Could you check a few things on this model? Use its own coordinates, in mm. Face numbers are marked on the shaded views. A direction names the side the tool comes from. Round coordinates to 2 decimals unless told otherwise and drop trailing zeros. Write each loop counter-clockwise with the first axis right and the second up, starting at its lowest first coordinate (ties: lowest second). Pieces come first, ordered by that corner, then holes. Notation, with made-up numbers: (-19.75, -34) -> (39.25, -34) arc R19 cw to (39.25, 2) -> close; hole circle Ø8 at (57, -35). An arc over 180 degrees is marked (long way). One line per question, with ' | ' between items. Start each with the question number.
1. For the marked faces 5, 6 and 7, which set-ups out of +Z, -Z, +X, -X, +Y, -Y let a thin tool reach every point of the face, with its end or its side?
2. Imagine slicing it at D-D, the plane y = 18.5. List the corners of the cut face in (x, z) for me, and give its area (3 significant figures).
3. Thinking about a two-plate mould opening in Z: for the marked faces 1, 2, 3 and 4, which applies, released by +Z, released by -Z, zero draft, split by the parting line, or undercut?
4. Imagine slicing it at C-C, the plane x = -19. List the corners of the cut face in (y, z) for me.
5. Imagine slicing it at B-B, the plane z = 6.5. State how many separate pieces and enclosed holes the cut face has, and give its area (3 significant figures).
6. For pin 1 Ø5.5 at (x, z) = (-19.5, 8) entering from +Y; pin 2 Ø3 at (x, z) = (5, 7.5) entering from +Y; pin 3 Ø5 at (x, y) = (0, -5) entering from +Z, each with a flat end and sliding along its axis, tell me the tip position at first contact or that it passes through.
7. If I drill on line 1 along Y through (x, z) = (0, 7); line 2 along Y through (x, z) = (0, 14.35); line 3 along X through (y, z) = (6.5, 10.25), over which ranges is the centre line in solid material (lowest first)? Write a range as [from, to].
8. Imagine slicing it at A-A, the plane y = -23.5. List the corners of the cut face in (x, z) for me.
from build123d import *

# Parameters (mm, degrees)
BOSS_EXTRUDE1_DEPTH = 15
CUT_EXTRUDE1_REACH  = 57
SKETCH2_R           = 2.25
SKETCH3_R           = 5.54
CUT_EXTRUDE2_DEPTH  = 21
SKETCH4_W           = 24
SKETCH4_H           = 7
CUT_EXTRUDE3_DEPTH  = 29
CUT_EXTRUDE4_REACH  = 17
CUT_EXTRUDE5_DEPTH  = 1.5
SKETCH7_R           = 3.25
BOSS_EXTRUDE2_DEPTH = 13.5
CUT_EXTRUDE6_REACH  = 15.5
SKETCH8_R           = 1.5
SKETCH9_R           = 2.5
CUT_EXTRUDE7_DEPTH  = 12
SKETCH10_R          = 0.48
BOSS_EXTRUDE3_DEPTH = 1.5


with BuildPart() as part:
    # Sketch1 → Boss-Extrude1 (new body)
    with BuildSketch(Plane.XY):
        with BuildLine():
            Line((25, 0), (25, -30))
            Line((25, -30), (-25, -30))
            Line((-25, -30), (-25, 0))
            ThreePointArc((-25, 0), (0, 25), (25, 0))
        make_face()
    extrude(amount=BOSS_EXTRUDE1_DEPTH)

    # Sketch2 → Cut-Extrude1 (cut, up to next)
    with BuildSketch(Plane.XZ.offset(30), mode=Mode.PRIVATE) as cut_extrude1_sk1:
        with Locations((-19, 7.5)):
            Circle(SKETCH2_R)
    cut_extrude1_tool1 = extrude(cut_extrude1_sk1.sketch, amount=-CUT_EXTRUDE1_REACH, mode=Mode.PRIVATE) & part.part
    add(cut_extrude1_tool1.solids().sort_by_distance((-19, -30, 7.5))[0], mode=Mode.SUBTRACT)
    # Sketch2 → Cut-Extrude1 (cut, up to next)
    with BuildSketch(Plane.XZ.offset(30), mode=Mode.PRIVATE) as cut_extrude1_sk2:
        with Locations((19, 7.5)):
            Circle(SKETCH2_R)
    cut_extrude1_tool2 = extrude(cut_extrude1_sk2.sketch, amount=-CUT_EXTRUDE1_REACH, mode=Mode.PRIVATE) & part.part
    add(cut_extrude1_tool2.solids().sort_by_distance((19, -30, 7.5))[0], mode=Mode.SUBTRACT)

    # Sketch3 → Cut-Extrude2 (cut)
    with BuildSketch(Plane(origin=(0, 24.127056635, 0), x_dir=(1, 0, 0), z_dir=(0, 1, 0))):
        with Locations((19, -7.5)):
            Circle(SKETCH3_R)
        with Locations((-19, -7.5)):
            Circle(SKETCH3_R)
    extrude(amount=-CUT_EXTRUDE2_DEPTH, mode=Mode.SUBTRACT)

    # Sketch4 → Cut-Extrude3 (cut)
    with BuildSketch(Plane.XZ.offset(30)):
        with Locations((0, 7.5)):
            Rectangle(SKETCH4_W, SKETCH4_H)
    extrude(amount=-CUT_EXTRUDE3_DEPTH, mode=Mode.SUBTRACT)

    # Sketch5 → Cut-Extrude4 (cut, up to next)
    with BuildSketch(Plane.XY.offset(15), mode=Mode.PRIVATE) as cut_extrude4_sk1:
        with BuildLine():
            Line((11.251747285, -5), (15, -5))
            ThreePointArc((15, -5), (0, -20), (-15, -5))
            ThreePointArc((-15, -5), (-13.858192988, 0.740251485), (-10.606601718, 5.606601718))
            Line((-10.606601718, 5.606601718), (-7.956186805, 2.956186805))
            ThreePointArc((-7.956186805, 2.956186805), (-10.395259022, -0.694142729), (-11.251747285, -5))
            ThreePointArc((-11.251747285, -5), (0, -16.251747285), (11.251747285, -5))
        make_face()
    cut_extrude4_tool1 = extrude(cut_extrude4_sk1.sketch, amount=-CUT_EXTRUDE4_REACH, mode=Mode.PRIVATE) & part.part
    add(cut_extrude4_tool1.solids().sort_by_distance((13.125874, -5.394423, 15))[0], mode=Mode.SUBTRACT)

    # Sketch6 → Cut-Extrude5 (cut)
    with BuildSketch(Plane.XY.offset(15)):
        with BuildLine():
            Line((0.541549319, -1.795436951), (14.169837516, 1.800031788))
            ThreePointArc((14.169837516, 1.800031788), (16.028383105, 0.812877901), (15.18982596, -1.117274015))
            Line((15.18982596, -1.117274015), (2.352905683, -7.241948894))
            ThreePointArc((2.352905683, -7.241948894), (-3.083924533, -6.02562638), (0.541549319, -1.795436951))
        make_face()
    extrude(amount=-CUT_EXTRUDE5_DEPTH, mode=Mode.SUBTRACT)

    # Sketch7 → Boss-Extrude2 (add)
    with BuildSketch(Plane.XY.offset(13.5)):
        with Locations((0, -5)):
            Circle(SKETCH7_R)
    extrude(amount=-BOSS_EXTRUDE2_DEPTH)

    # Sketch8 → Cut-Extrude6 (cut, up to next)
    with BuildSketch(Plane.XY.offset(13.5), mode=Mode.PRIVATE) as cut_extrude6_sk1:
        with Locations((0, -5)):
            Circle(SKETCH8_R)
    cut_extrude6_tool1 = extrude(cut_extrude6_sk1.sketch, amount=-CUT_EXTRUDE6_REACH, mode=Mode.PRIVATE) & part.part
    add(cut_extrude6_tool1.solids().sort_by_distance((0, -5, 13.5))[0], mode=Mode.SUBTRACT)

    # Sketch9 → Cut-Extrude7 (cut)
    with BuildSketch(Plane(origin=(0, 0, 0), x_dir=(-1, 0, 0), z_dir=(0, 0, -1))):
        with Locations((0, -5)):
            Circle(SKETCH9_R)
    extrude(amount=-CUT_EXTRUDE7_DEPTH, mode=Mode.SUBTRACT)

    # Sketch10 → Boss-Extrude3 (add)
    with BuildSketch(Plane.XY.offset(13.5)):
        with Locations((14.565235622, 0.301312222)):
            Circle(SKETCH10_R)
        with Locations((12.477655938, -0.392957944)):
            Circle(SKETCH10_R)
        with Locations((10.390076254, -1.087228109)):
            Circle(SKETCH10_R)
        with Locations((8.30249657, -1.781498274)):
            Circle(SKETCH10_R)
        with Locations((6.214916885, -2.475768439)):
            Circle(SKETCH10_R)
        with Locations((4.127337201, -3.170038604)):
            Circle(SKETCH10_R)
    extrude(amount=BOSS_EXTRUDE3_DEPTH)


solid = part.part
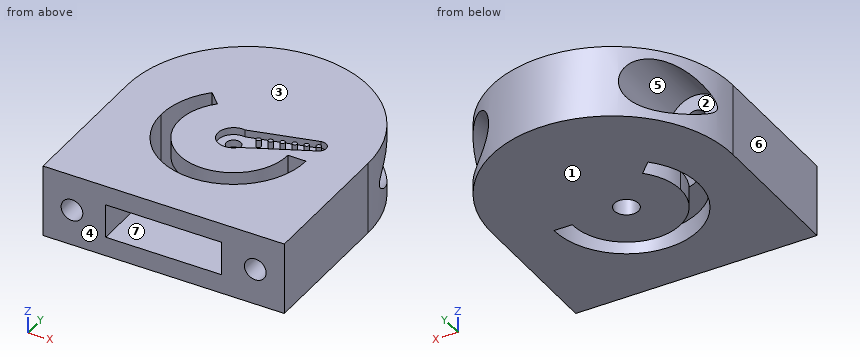
Geometry results:
1) face 5: +Y | face 6: +Z, -Z, -X, +Y, -Y | face 7: -Y
2) outline: (-16.82, 0) -> (16.82, 0) -> (16.82, 2.41) arc R5.54 cw to (16.82, 12.59) -> (16.82, 15) -> (-16.82, 15) -> (-16.82, 12.59) arc R5.54 cw to (-16.82, 2.41) -> close | area: 455 mm2
3) face 1: released by -Z | face 2: undercut | face 3: released by +Z | face 4: zero draft
4) outline: (-30, 0) -> (16.25, 0) -> (16.25, 1.96) -> (3.13, 1.96) -> (3.13, 5.25) -> (-30, 5.25) -> close; (-30, 9.75) -> (3.13, 9.75) -> (3.13, 13.04) -> (16.25, 13.04) -> (16.25, 15) -> (-30, 15) -> close
5) separate pieces: 4 | enclosed holes: 1 | area: 1,190 mm2
6) pin 1: stops at y = 3.13 | pin 2: stops at y = 24.75 | pin 3: stops at z = 13.5
7) line 1: y = [-8.25, -7.5], [-2.5, -1.75], [-1, 25] | line 2: y = [-30, -20], [-16.25, -8.25], [-1.75, 25] | line 3: x = [-24.14, -23.81], [-14.19, 14.19], [23.81, 24.14]
8) outline: (-25, 0) -> (25, 0) -> (25, 15) -> (-25, 15) -> close; hole circle Ø4.5 at (-19, 7.5); hole (-12, 4) -> (12, 4) -> (12, 11) -> (-12, 11) -> close; hole circle Ø4.5 at (19, 7.5)
